For this review, take the finished solid that the model builds, in its own axes (mm). Face numbers are marked on the shaded views. A direction names the side the tool comes from. Round coordinates to 2 decimals unless told otherwise and drop trailing zeros. Order: outer loops, then holes, each group sorted by start corner. A loop starts at its lowest first (then second) coordinate and runs counter-clockwise, first axis right, second up. Notation, with made-up numbers: (40.25, -4) -> (73.25, -4) arc R16 cw to (73.25, 10) -> close; hole circle Ø9 at (23.25, 55.25). An arc over 180 degrees is marked (long way). Put each result on its own line as item: value. Start each with the question number.
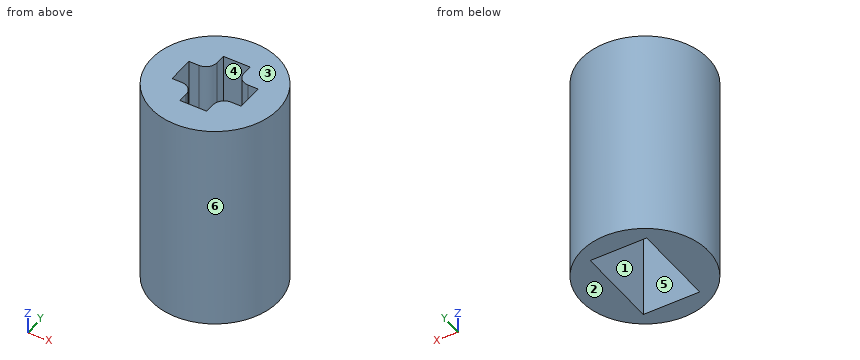
```python
from build123d import *

# Parameters (mm, degrees)
SKETCH1_R           = 4.5
BOSS_EXTRUDE1_DEPTH = 15
SKETCH2_W           = 4
SKETCH2_H           = 6
CUT_EXTRUDE1_DEPTH  = 7
CUT_EXTRUDE2_DEPTH  = 7
FILLET3_R           = 0.8


with BuildPart() as part:
    # Sketch1 → Boss-Extrude1 (new body)
    with BuildSketch(Plane.XY):
        Circle(SKETCH1_R)
    extrude(amount=BOSS_EXTRUDE1_DEPTH)

    # Sketch2 → Cut-Extrude1 (cut)
    with BuildSketch(Plane(origin=(0, 0, 0), x_dir=(-1, 0, 0), z_dir=(0, 0, -1))):
        Rectangle(SKETCH2_W, SKETCH2_H)
    extrude(amount=-CUT_EXTRUDE1_DEPTH, mode=Mode.SUBTRACT)

    # Sketch3 → Cut-Extrude2 (cut)
    with BuildSketch(Plane.XY.offset(15)):
        Polygon((-0.95, -0.95), (-0.95, -2.45), (0.95, -2.45), (0.95, -0.95), (2.45, -0.95), (2.45, 0.95), (0.95, 0.95), (0.95, 2.45), (-0.95, 2.45), (-0.95, 0.95), (-2.45, 0.95), (-2.45, -0.95), align=None)
    extrude(amount=-CUT_EXTRUDE2_DEPTH, mode=Mode.SUBTRACT)

    # Fillet3
    fillet3_edges = [part.edges().sort_by_distance(p)[0] for p in [
        (0.95, -0.95, 11.5),
        (-0.95, -0.95, 11.5),
        (-0.95, 0.95, 11.5),
        (0.95, 0.95, 11.5),
    ]]
    fillet(fillet3_edges, radius=FILLET3_R)


solid = part.part
```
Item 1: Consider section A-A, the plane z = 2.5. Write out the cut boundary in (x, y), plus the area to 3 significant figures.
Item 2: Tool access review of the marked faces 1 and 2: name each direction out of +Z, -Z, +X, -X, +Y, -Y from which nothing blocks a thin tool from reaching the whole face with its end or side.
Item 3: Consider section D-D, the plane z = 12.5. Write out the cut boundary in (x, y), plus the area to 3 significant figures.
Item 4: Consider section C-C, the plane y = 0. Write out the cut boundary in (x, z), plus the area to 3 significant figures.
Item 5: Consider section B-B, the plane x = 0. Write out the cut boundary in (y, z), plus the area to 3 significant figures.
Item 6: For L1, parallel to X at y = 1.5, z = 5; L2, parallel to X at y = -1.75, z = 10; L3, parallel to Y at x = 0, z = 10.5, list the stretches that pass through material, from the lowest coordinate up.
Item 7: Mouldability with a two-part tool opening along X and no side actions: class the marked faces 3, 4, 5 and 6 as +X half, -X half, draft (parallel to the pull), parting line (faces both ways), or undercut.
Item 8: Insertion check: pin 1 Ø0.8 at (y, z) = (2, 13) entering from -X; pin 2 Ø0.6 at (x, z) = (-2, 12.5) entering from +Y; pin 3 Ø5 at (y, z) = (-1.5, 5) entering from +X; pin 4 Ø0.6 at (y, z) = (-2, 12) entering from +X. Each pin has a flat end and moves straight along its axis. Give the tip position at first contact, or say it passes through.
Evaluation:
1. outline: circle Ø9 at (0, 0); hole (-2, -3) -> (2, -3) -> (2, 3) -> (-2, 3) -> close
1. area: 39.6 mm^2
2. face 1: -Z
2. face 2: -Z, +X, -X, +Y, -Y
3. outline: circle Ø9 at (0, 0); hole (-2.45, -0.95) -> (-1.75, -0.95) arc R0.8 cw to (-0.95, -1.75) -> (-0.95, -2.45) -> (0.95, -2.45) -> (0.95, -1.75) arc R0.8 cw to (1.75, -0.95) -> (2.45, -0.95) -> (2.45, 0.95) -> (1.75, 0.95) arc R0.8 cw to (0.95, 1.75) -> (0.95, 2.45) -> (-0.95, 2.45) -> (-0.95, 1.75) arc R0.8 cw to (-1.75, 0.95) -> (-2.45, 0.95) -> close
3. area: 48.1 mm^2
4. outline: (-4.5, 0) -> (-2, 0) -> (-2, 7) -> (2, 7) -> (2, 0) -> (4.5, 0) -> (4.5, 15) -> (2.45, 15) -> (2.45, 8) -> (-2.45, 8) -> (-2.45, 15) -> (-4.5, 15) -> close
4. area: 72.7 mm^2
5. outline: (-4.5, 0) -> (-3, 0) -> (-3, 7) -> (3, 7) -> (3, 0) -> (4.5, 0) -> (4.5, 15) -> (2.45, 15) -> (2.45, 8) -> (-2.45, 8) -> (-2.45, 15) -> (-4.5, 15) -> close
5. area: 58.7 mm^2
6. L1: x = -4.24 to -2, 2 to 4.24
6. L2: x = -4.15 to -0.95, 0.95 to 4.15
6. L3: y = -4.5 to -2.45, 2.45 to 4.5
7. face 3: draft
7. face 4: undercut
7. face 5: undercut
7. face 6: parting line
8. pin 1: stops at x = -4.21
8. pin 2: stops at y = 4.17
8. pin 3: stops at x = 4.5
8. pin 4: stops at x = 4.17
